The drawing under review shows one solid part. Ordinate dimensions are in mm from its lowest x, y, z. Round coordinates to 2 decimals unless told otherwise and drop trailing zeros. Order: outer loops, then holes, each group sorted by start corner. A loop starts at its lowest first (then second) coordinate and runs counter-clockwise, first axis right, second up. Notation, with made-up numbers: (73, -11) -> (119, -11) arc R8 cw to (119, 1) -> close; hole circle Ø6 at (62.25, 1.25). An arc over 180 degrees is marked (long way). Put each result on its own line as item: value. Start each with the question number.
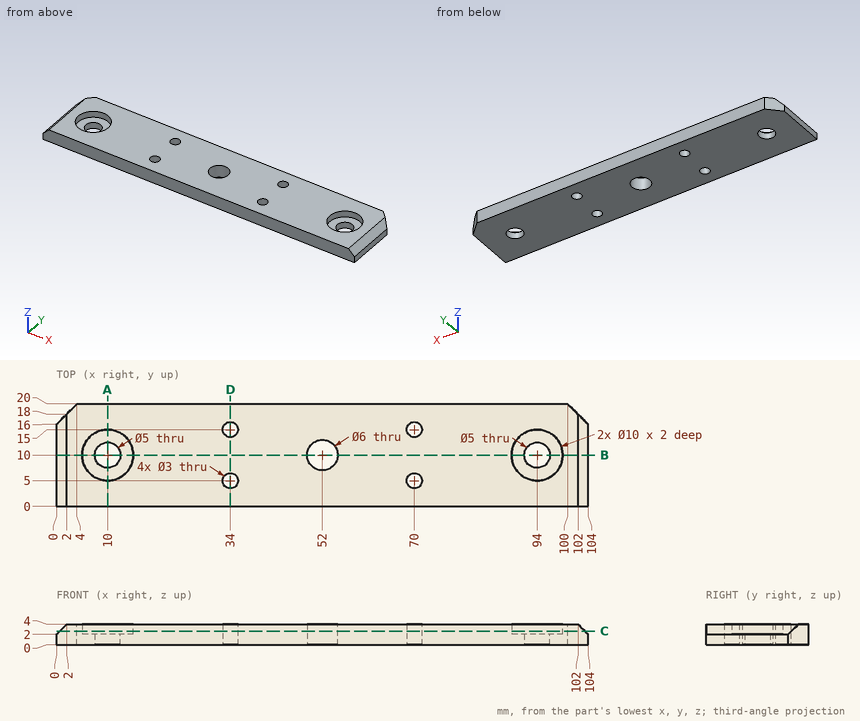
Item 1: Consider section A-A, the plane x = 10. Write out the cut boundary in (y, z), plus the area to 3 significant figures.
Item 2: Insertion check: pin 1 Ø5 at (x, y) = (93.5, 9.5) entering from +Z; pin 2 Ø1.5 at (y, z) = (9, 3.5) entering from +X. Each pin has a flat end and moves straight along its axis. Give the tip position at first contact, or say it passes through.
Item 3: For L1, parallel to X at y = 5, z = 1.8; L2, parallel to X at y = 10, z = 0.85; L3, parallel to Y at x = 10, z = 3.8, list the stretches that pass through material, from the lowest coordinate up.
Item 4: Consider section D-D, the plane x = 34. Write out the cut boundary in (y, z), plus the area to 3 significant figures.
Item 5: Consider section B-B, the plane y = 10. Write out the cut boundary in (x, z), plus the area to 3 significant figures.
Item 6: Consider section C-C, the plane z = 2.65. Write out the cut boundary in (x, y).
Evaluation:
1. outline: (0, 0) -> (7.5, 0) -> (7.5, 2) -> (5, 2) -> (5, 4) -> (0, 4) -> close; (12.5, 0) -> (20, 0) -> (20, 4) -> (15, 4) -> (15, 2) -> (12.5, 2) -> close
1. area: 50.0 mm^2
2. pin 1: stops at z = 2
2. pin 2: stops at x = 103.25
3. L1: x = 0 to 32.5, 35.5 to 68.5, 71.5 to 104
3. L2: x = 0 to 7.5, 12.5 to 49, 55 to 91.5, 96.5 to 104
3. L3: y = 0 to 5, 15 to 20
4. outline: (0, 0) -> (3.5, 0) -> (3.5, 4) -> (0, 4) -> close; (6.5, 0) -> (13.5, 0) -> (13.5, 4) -> (6.5, 4) -> close; (16.5, 0) -> (20, 0) -> (20, 4) -> (16.5, 4) -> close
4. area: 56.0 mm^2
5. outline: (0, 0) -> (7.5, 0) -> (7.5, 2) -> (5, 2) -> (5, 4) -> (2, 4) -> (0, 2) -> close; (12.5, 0) -> (49, 0) -> (49, 4) -> (15, 4) -> (15, 2) -> (12.5, 2) -> close; (55, 0) -> (91.5, 0) -> (91.5, 2) -> (89, 2) -> (89, 4) -> (55, 4) -> close; (96.5, 0) -> (104, 0) -> (104, 2) -> (102, 4) -> (99, 4) -> (99, 2) -> (96.5, 2) -> close
5. area: 328 mm^2
6. outline: (0.65, 0) -> (103.35, 0) -> (103.35, 16.65) -> (100, 20) -> (4, 20) -> (0.65, 16.65) -> close; hole circle Ø10 at (10, 10); hole circle Ø3 at (34, 5); hole circle Ø3 at (34, 15); hole circle Ø6 at (52, 10); hole circle Ø3 at (70, 5); hole circle Ø3 at (70, 15); hole circle Ø10 at (94, 10)
